from build123d import *

# Parameters (mm, degrees)
F0_W          = 2006.6
F0_H          = 1524
F1_DEPTH      = 254
F4_DEPTH      = 914.4
F5_DEPTH      = 88.901
F6_DEPTH      = 88.901
F3_W          = 457.2
F3_H          = 457.2
F7_DEPTH      = 2006.6
F8_DEPTH      = 914.4
F8_DEPTH_BACK = 914.4
F9_W          = 1828.8
F9_H          = 317.5
F10_DEPTH     = 355.6
F11_W         = 1828.8
F11_H         = 38.1
F12_DEPTH     = 188.9265486726
F13_R         = 57.15
F14_DEPTH     = 88.901
F15_DEPTH     = 152.4


with BuildPart() as f1:
    # F0 (on Top) → F1 (new body)
    with BuildSketch(Plane.XY):
        Rectangle(F0_W, F0_H)
    extrude(amount=F1_DEPTH)

    # F2 (on Right) → F4 (cut, symmetric)
    with BuildSketch(Plane.YZ):
        Polygon((673.1, 254), (-762, 254), (673.1, 88.9), align=None)
        Polygon((673.1, 0), (-762, 165.1), (-762, 0), align=None)
    extrude(amount=F4_DEPTH, both=True, mode=Mode.SUBTRACT)

    # F5 (cut, through all): a face of the model
    f5_faces = [f1.faces().sort_by_distance(p)[0] for p in [
        (-914.4, -283.6333333333, 55.0333333333),
    ]]
    extrude(f5_faces, amount=-F5_DEPTH, mode=Mode.SUBTRACT)

    # F6 (cut, through all): a face of the model
    f6_faces = [f1.faces().sort_by_distance(p)[0] for p in [
        (914.4, -283.6333333333, 55.0333333333),
    ]]
    extrude(f6_faces, amount=-F6_DEPTH, mode=Mode.SUBTRACT)

    # F3 (on face) → F7 (join, through all)
    with BuildSketch(Plane(origin=(-1003.3, 0, 0), x_dir=(0, -1, 0), z_dir=(-1, 0, 0))):
        with Locations((-533.4, 25.4)):
            Rectangle(F3_W, F3_H)
    extrude(amount=-F7_DEPTH)

    # F2 (on Right) → F8 (cut, two sides)
    with BuildSketch(Plane.YZ) as f8_sk:
        Polygon((673.1, 254), (-762, 254), (673.1, 88.9), align=None)
    extrude(amount=-F8_DEPTH, mode=Mode.SUBTRACT)
    extrude(f8_sk.sketch, amount=F8_DEPTH_BACK, mode=Mode.SUBTRACT)

    # F9 (on face) → F10 (cut, through all)
    with BuildSketch(Plane.XY.offset(254)):
        with Locations((0, 514.35)):
            Rectangle(F9_W, F9_H)
    extrude(amount=-F10_DEPTH, mode=Mode.SUBTRACT)

    # F11 (on face) → F12 (join, through all)
    with BuildSketch(Plane.XY.offset(-101.6)):
        with Locations((0, 654.05)):
            Rectangle(F11_W, F11_H)
        with Locations((0, 374.65)):
            Rectangle(F11_W, F11_H)
    extrude(amount=F12_DEPTH)

    # F13 (on face) → F14 (cut, through all)
    with BuildSketch(Plane.YZ.offset(-914.4)):
        with Locations((514.35, -44.45)):
            Circle(F13_R)
    extrude(amount=-F14_DEPTH, mode=Mode.SUBTRACT)

    # F15 (add): a face of the model
    f15_faces = [f1.faces().sort_by_distance(p)[0] for p in [
        (0, -762, 209.55),
    ]]
    extrude(f15_faces, amount=F15_DEPTH)


solid = f1.part
Read the model definition and answer for the solid it produces. Units are mm, in the model's axes. A direction names the side the tool comes from. Coordinates: 2 decimals unless noted, no trailing zeros. Loops run counter-clockwise (first coordinate to the right, second up) from the corner with the lowest first, then second, coordinate; pieces in that order, holes last. Notation, with made-up numbers: (41.5, -30.75) - (93.5, -30.75) arc R15 ccw to (93.5, -8.75) - close; hole circle Ø3 at (-1.5, -7.75). An arc over 180 degrees is marked (long way). Answer in a Markdown table with one row per item.
Q1. Find section C-C on x = -549.5. Write down the section's boundary in (y, z).
Here are the results:
| item | result |
|---|---|
| outline | (-914.4, 165.1) - (-762, 165.1) - (304.8, 42.37) - (304.8, -203.2) - (762, -203.2) - (762, 254) - (673.1, 254) - (673.1, 87.33) - (635, 87.33) - (635, -101.6) - (393.7, -101.6) - (393.7, 87.33) - (355.6, 87.33) - (355.6, 125.43) - (-762, 254) - (-914.4, 254) - close |
Q2. Find section D-D on z = 226. Write down the section's boundary in (x, y), plus the area to 3 significant figures.
Here are the results:
| item | result |
|---|---|
| outline | (-1003.3, -914.4) - (1003.3, -914.4) - (1003.3, 762) - (-1003.3, 762) - close; hole (-914.4, -518.62) - (914.4, -518.62) - (914.4, 673.1) - (-914.4, 673.1) - close |
| area | 1,180,000 mm^2 |
Q3. For faces 1 (the flat face through (-13, 673.1, 169)), 2 (the flat face through (-14, 762, 22)), 3 (the flat face through (14, -837, 165.1)), determine the directions among +Z, -Z, +X, -X, +Y, -Y from which every point of the face is accessible in a straight line to the end or side of a thin tool.
Here are the results:
| item | result |
|---|---|
| face 1 | +Z |
| face 2 | +Z, -Z, +X, -X, +Y |
| face 3 | -Z, +X, -X, -Y |
Q4. Find section B-B on z = -44.45. Write down the section's boundary in (x, y), plus the area to 3 significant figures.
Here are the results:
| item | result |
|---|---|
| outline | (-1003.3, 304.8) - (1003.3, 304.8) - (1003.3, 762) - (-1003.3, 762) - (-1003.3, 571.5) - (-914.4, 571.5) - (-914.4, 635) - (914.4, 635) - (914.4, 393.7) - (-914.4, 393.7) - (-914.4, 457.2) - (-1003.3, 457.2) - close |
| area | 466,000 mm^2 |
Q5. Find section A-A on y = 427. Write down the section's boundary in (x, z), plus the area to 3 significant figures.
Here are the results:
| item | result |
|---|---|
| outline | (-1003.3, -203.2) - (1003.3, -203.2) - (1003.3, 254) - (914.4, 254) - (914.4, -101.6) - (-914.4, -101.6) - (-914.4, 254) - (-1003.3, 254) - close |
| area | 267,000 mm^2 |
Q6. Straight lines are drawn through the part: line 1 along X through (y, z) = (167, 148); line 2 along Y through (x, z) = (-962, -44); line 3 along Z through (x, y) = (-983.5, 514.35). For each, find the intervals that lie inside material, in ascending order. Write a range as [from, to].
Here are the results:
| item | result |
|---|---|
| line 1 | x = [-1003.3, -914.4], [914.4, 1003.3] |
| line 2 | y = [304.8, 457.2], [571.5, 762] |
| line 3 | z = [-203.2, -101.6], [12.7, 254] |
Q7. The mould has two halves that part along Z. Classify faces 4 (the flat face through (-13, 516, -101.6)), 5 (the flat face through (14.046, -221.132, 102.876)), 6 (the cylindrical face through (-958.23, 567.14, -66.34)), 7 (the flat face through (-1003.3, 122, 73)): pulls with the +Z half, pulls with the -Z half, needs draft (parallel to the pull), parting line crosses it, or undercut.
Here are the results:
| item | result |
|---|---|
| face 4 | pulls with the +Z half |
| face 5 | pulls with the -Z half |
| face 6 | undercut |
| face 7 | needs draft |
Q8. Given P1, Ø12, axis at x = 714.5, y = 81.5, coming from the +Z side; P2, Ø1.5, axis at x = 377.5, y = 369, coming from the +Z side, each flat-ended and moving along its own axis, determine where each tip first touches the part or whether it passes through.
Here are the results:
| item | result |
|---|---|
| P1 | stops at z = 157.65 |
| P2 | stops at z = 87.33 |
